Verification items for this drawing (mm, ordinates from the low corner). Round coordinates to 2 decimals unless told otherwise and drop trailing zeros. Order: outer loops, then holes, each group sorted by start corner. A loop starts at its lowest first (then second) coordinate and runs counter-clockwise, first axis right, second up. Notation, with made-up numbers: (43.5, 36.25) - (93.5, 36.25) arc R19 ccw to (93.5, 58.25) - close; hole circle Ø2 at (80, 67.25). An arc over 180 degrees is marked (long way). Return JSON: item names as keys, results as strings. Group by question number.
Q1. Sectioned sample at A-A, the plane z = 5.75. Record the cut outline in (x, y) (3 decimals), then the cut area to 3 significant figures.
Q2. Draft check along X on the marked faces 1, 2 and 3. Enter one of: pulls with the +X half, pulls with the -X half, needs draft (parallel to the pull), parting line crosses it, or undercut.
Q3. Gauge pin test, flat ends, axial feed: pin 1 Ø1.5 at (y, z) = (47, 3.5) entering from -X; pin 2 Ø3 at (y, z) = (15.5, 2) entering from -X; pin 3 Ø4 at (y, z) = (41.5, 2.5) entering from +X. Record the tip position at first contact, or that the pin passes through.
Q4. Material ranges on line 1 along Y through (x, z) = (33.5, 10.75) (1 decimal); line 2 along X through (y, z) = (36, 1.25); line 3 along Y through (x, z) = (22, 1), recorded low to high.
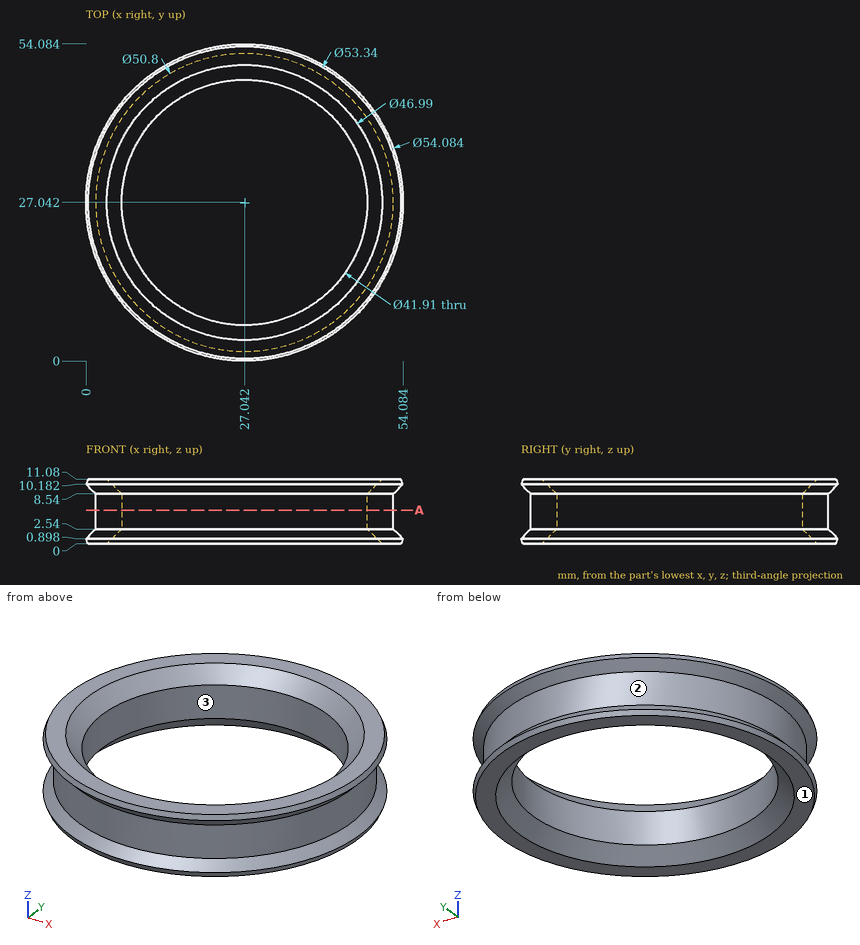
Reply:
{
 "1": {"outline": "circle Ø50.8 at (27.042, 27.042); hole circle Ø41.91 at (27.042, 27.042)", "area": "647 mm^2"},
 "2": {"face 1": "needs draft", "face 2": "parting line crosses it", "face 3": "undercut"},
 "3": {"pin 1": "x = 10.42", "pin 2": "x = 2.13", "pin 3": "x = 50.61"},
 "4": {"line 1": "1 to 4.8, 49.3 to 53.1", "line 2": "1.9 to 6.68, 47.4 to 52.18", "line 3": "0.58 to 5.12, 48.96 to 53.51"}
}
